CAD build for the part. Positions are in the model's coordinates, mm. Give positions to 0.01 mm unless a question says otherwise; leave off trailing zeros. Order: outer loops, then holes, each group sorted by start corner. A loop starts at its lowest first (then second) coordinate and runs counter-clockwise, first axis right, second up. Notation, with made-up numbers: (55, 14) -> (100, 14) arc R29 cw to (100, 47) -> close; hole circle Ø9 at (11.5, 44). An arc over 180 degrees is marked (long way). Answer as CSV lines item,"result".
```python
from build123d import *

# Parameters (mm, degrees)
EXTRUDE_3_DEPTH = 1


with BuildPart() as part:
    # 草图1 → 凸台-拉伸3 (new body)
    with BuildSketch(Plane.XY):
        with BuildLine():
            ThreePointArc((-0.3, 4), (0, 4.3), (0.3, 4))
            Line((0.3, 4), (0.888888889, 4))
            ThreePointArc((0.888888889, 4), (0, 4.888888889), (-0.888888889, 4))
            Line((-0.888888889, 4), (-0.3, 4))
        make_face()
        with BuildLine():
            Line((0.888888889, 4), (0.3, 4))
            ThreePointArc((0.3, 4), (0, 3.7), (-0.3, 4))
            Line((-0.3, 4), (-0.888888889, 4))
            ThreePointArc((-0.888888889, 4), (0, 3.111111111), (0.888888889, 4))
        make_face()
        with BuildLine():
            Line((0.888888889, -4), (0.888888889, 4))
            ThreePointArc((0.888888889, 4), (0, 3.111111111), (-0.888888889, 4))
            Line((-0.888888889, 4), (-0.888888889, -4))
            ThreePointArc((-0.888888889, -4), (0, -3.111111111), (0.888888889, -4))
        make_face()
        with BuildLine():
            ThreePointArc((-0.888888889, -4), (0, -4.888888889), (0.888888889, -4))
            Line((0.888888889, -4), (0.3, -4))
            ThreePointArc((0.3, -4), (0, -4.3), (-0.3, -4))
            Line((-0.3, -4), (-0.888888889, -4))
        make_face()
        with BuildLine():
            Line((0.3, -4), (0.888888889, -4))
            ThreePointArc((0.888888889, -4), (0, -3.111111111), (-0.888888889, -4))
            Line((-0.888888889, -4), (-0.3, -4))
            ThreePointArc((-0.3, -4), (0, -3.7), (0.3, -4))
        make_face()
    extrude(amount=EXTRUDE_3_DEPTH)


solid = part.part
```
1) Band-saw the part on C-C, the plane x = 0.65. Write the cut outline in (y, z).
Data:
outline,"(-4.61, 0) -> (4.61, 0) -> (4.61, 1) -> (-4.61, 1) -> close"
2) Band-saw the part on A-A, the plane x = 0. Write the cut outline in (y, z).
Data:
outline,"(-4.89, 0) -> (-4.3, 0) -> (-4.3, 1) -> (-4.89, 1) -> close; (-3.7, 0) -> (3.7, 0) -> (3.7, 1) -> (-3.7, 1) -> close; (4.3, 0) -> (4.89, 0) -> (4.89, 1) -> (4.3, 1) -> close"
3) Wall check: line 1 along Y through (x, z) = (0, 0.5); line 2 along X through (y, z) = (-4, 0.7); line 3 along Y through (x, z) = (0.4, 0.8). Give the ranges that are in metal, low to high. Write a range as [from, to].
Data:
line 1,"y = [-4.89, -4.3], [-3.7, 3.7], [4.3, 4.89]"
line 2,"x = [-0.89, -0.3], [0.3, 0.89]"
line 3,"y = [-4.79, 4.79]"
4) Band-saw the part on B-B, the plane z = 0.7. Write the cut outline in (x, y).
Data:
outline,"(-0.89, -4) arc R0.89 ccw to (0.89, -4) -> (0.89, 4) arc R0.89 ccw to (-0.89, 4) -> close; hole circle Ø0.6 at (0, -4); hole circle Ø0.6 at (0, 4)"
